Work out the finished part from the listing and answer in its coordinate system (mm). A direction names the side the tool comes from. Give positions to 0.01 mm unless a question says otherwise; leave off trailing zeros. Loops run counter-clockwise (first coordinate to the right, second up) from the corner with the lowest first, then second, coordinate; pieces in that order, holes last. Notation, with made-up numbers: (39, 82.25) - (95, 82.25) arc R11 ccw to (95, 95.25) - close; hole circle Ø10 at (-13, 19.5). An arc over 180 degrees is marked (long way). Use CSV: the item, a comma, the result in double quotes.
from build123d import *

# Parameters (mm, degrees)
F1_DEPTH = 5


with BuildPart() as f1:
    # F0 (on Top) → F1 (new body)
    with BuildSketch(Plane.XY):
        with BuildLine():
            Line((-65.410274, 44.314684), (-68.597218, 44.329395))
            ThreePointArc((-68.597218, 44.329395), (-63.681228, 39.740166), (-58.723081, 44.283817))
            Line((-58.723081, 44.283817), (-58.723081, 47.183014))
            Line((-58.723081, 47.183014), (-58.70503, 51.093523))
            Line((-58.70503, 51.093523), (-58.70503, 53.350328))
            Line((-58.70503, 53.350328), (-61.986422, 53.365474))
            Line((-61.986422, 53.365474), (-61.986422, 51.093523))
            Line((-61.986422, 51.093523), (-61.986422, 44.29888))
            ThreePointArc((-61.986422, 44.29888), (-63.70606, 42.635903), (-65.410274, 44.314684))
        make_face()
    extrude(amount=F1_DEPTH)


solid = f1.part
Item 1: Find the intervals of material crossed by line 1 (X direction, y = 47, z = 3.85); line 2 (X direction, y = 44, z = 4.5); line 3 (Y direction, x = -63.75, z = 4.05), in increasing order.
Determined:
line 1,"x = -61.99 to -58.72"
line 2,"x = -68.56 to -65.37, -62.02 to -58.75"
line 3,"y = 39.74 to 42.64"
Item 2: Given P1, Ø2.5, axis at y = 46, z = 3, coming from the +X side; P2, Ø1, axis at x = -60.5, z = 4, coming from the +Y side, each flat-ended and moving along its own axis, determine where each tip first touches the part or whether it passes through.
Determined:
P1,"stops at x = -58.72"
P2,"stops at y = 53.36"
Item 3: A cutting plane is placed at A-A on y = 44. Determine the outline of the cut face in (x, z), and give its area (3 significant figures).
Determined:
outline,"(-68.56, 0) - (-65.37, 0) - (-65.37, 5) - (-68.56, 5) - close; (-62.02, 0) - (-58.75, 0) - (-58.75, 5) - (-62.02, 5) - close"
area,"32.3 mm²"
Item 4: For faces 4 (the cylindrical face through (-63.78, 39.74, 2.46)), 5 (the flat face through (-58.723, 46, 2)), determine the directions among +Z, -Z, +X, -X, +Y, -Y from which every point of the face is accessible in a straight line to the end or side of a thin tool.
Determined:
face 4,"+Z, -Z, -Y"
face 5,"+Z, -Z, +X, -Y"
Item 5: A cutting plane is placed at C-C on x = -66.5. Determine the outline of the cut face in (y, z).
Determined:
outline,"(40.64, 0) - (44.32, 0) - (44.32, 5) - (40.64, 5) - close"
Item 6: A cutting plane is placed at B-B on z = 1.6. Determine the outline of the cut face in (x, y).
Determined:
outline,"(-68.6, 44.33) arc R4.95 ccw to (-58.72, 44.28) - (-58.72, 47.18) - (-58.71, 51.09) - (-58.71, 53.35) - (-61.99, 53.37) - (-61.99, 44.3) arc R1.71 cw to (-65.41, 44.31) - close"
Item 7: The mould has two halves that part along X. Classify faces 1 (the flat face through (-61.5, 45.1, 0)), 2 (the cylindrical face through (-63.669, 42.636, 2.465)), 3 (the flat face through (-58.705, 52, 2)): pulls with the +X half, pulls with the -X half, needs draft (parallel to the pull), parting line crosses it, or undercut.
Determined:
face 1,"needs draft"
face 2,"undercut"
face 3,"pulls with the +X half"
Item 8: A cutting plane is placed at D-D on y = 45.5. Determine the outline of the cut face in (x, z).
Determined:
outline,"(-61.99, 0) - (-58.72, 0) - (-58.72, 5) - (-61.99, 5) - close"
